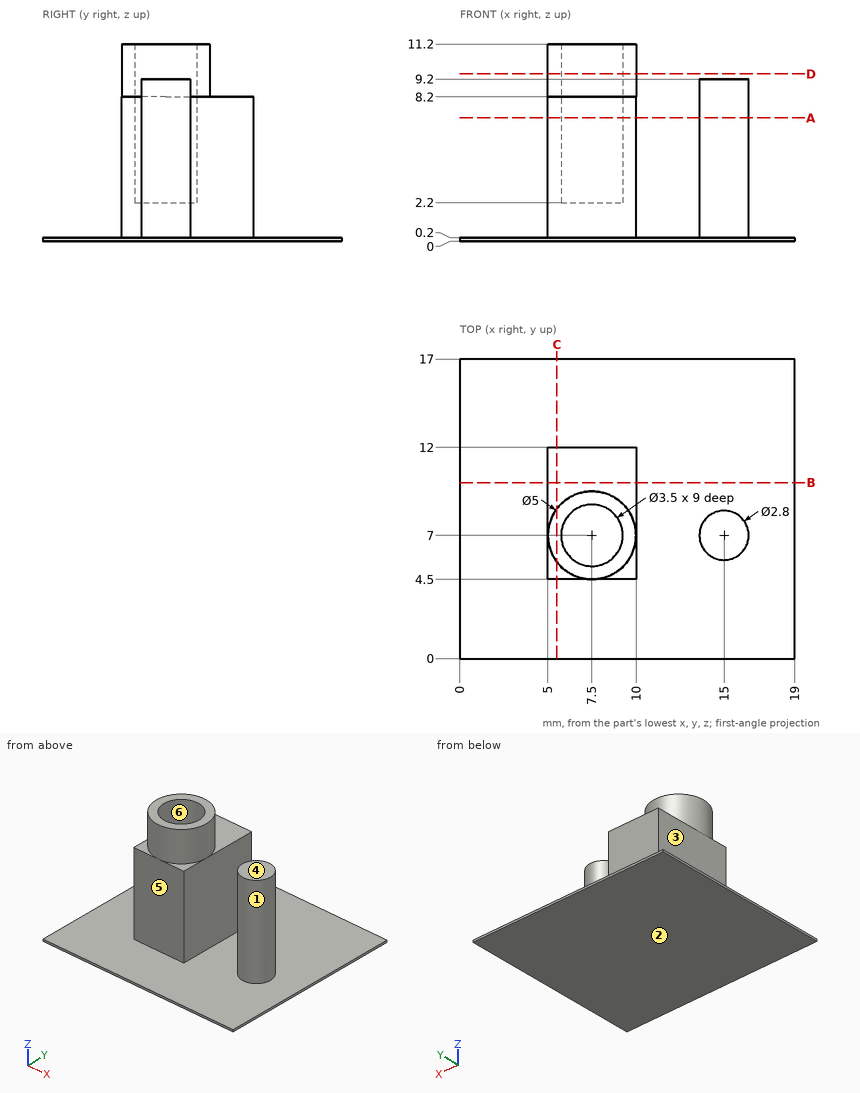
Could you check a few things on this drawing? It's one solid part, dimensions in mm from its lowest x, y, z. A direction names the side the tool comes from. Round coordinates to 2 decimals unless told otherwise and drop trailing zeros. Loops run counter-clockwise (first coordinate to the right, second up) from the corner with the lowest first, then second, coordinate; pieces in that order, holes last. Notation, with made-up numbers: M 50,68.25 L 107,68.25 A19 cw 107,73.25 Z; hole C 18,67 d5. An arc over 180 degrees is marked long. Write each question's results on one line, items separated by ' | '. Start each with the question number.
(1) If I drill on probe 1 along Y at (x, z) = (7.5, 7); probe 2 along Z at (x, y) = (5.75, 9.25); probe 3 along Z at (x, y) = (6.75, 2.25), over which ranges is the centre line in solid material (lowest first)? Write a range as from..to.
(2) I want a section at D-D (z = 9.5). Please give me the cut outline in (x, y), then the cut area to 3 significant figures.
(3) I want a section at B-B (y = 10). Please give me the cut outline in (x, z), then the cut area to 3 significant figures.
(4) Thinking about a two-plate mould opening in X: for the marked faces 1, 2 and 3, which applies, pulls with the +X half, pulls with the -X half, needs draft (parallel to the pull), parting line crosses it, or undercut?
(5) I want a section at C-C (x = 5.5). Please give me the cut outline in (y, z), then the cut area to 3 significant figures.
(6) I want a section at A-A (z = 7). Please give me the cut outline in (x, y), then the cut area to 3 significant figures.
(7) On a 3-axis mill with a long thin cutter (end or side, diameter ignored), from which of +Z, -Z, +X, -X, +Y, -Y can I reach the whole of each face in a straight line? I mean the marked faces 4, 5 and 6. Say none if no direction works.
(8) Will these pins go through, and if not, where does the flat tip stop? P1, Ø5, axis at x = 4, z = 3.5, coming from the -Y side; P2, Ø3, axis at y = 14, z = 3.5, coming from the +X side; P3, Ø1.5, axis at x = 7.5, z = 3, coming from the +Y side; P4, Ø2, axis at y = 8.5, z = 6, coming from the -X side.
Solved:
1) probe 1: y = 4.5..5.25, 8.75..12 | probe 2: z = 0..8.2 | probe 3: z = 0..0.2
2) outline: C 7.5,7 d5; hole C 7.5,7 d3.5 | area: 10.0 mm²
3) outline: M 0,0 L 19,0 L 19,0.2 L 10,0.2 L 10,8.2 L 5,8.2 L 5,0.2 L 0,0.2 Z | area: 43.8 mm²
4) face 1: undercut | face 2: needs draft | face 3: pulls with the -X half
5) outline: M 0,0 L 17,0 L 17,0.2 L 12,0.2 L 12,8.2 L 8.5,8.2 L 8.5,11.2 L 5.5,11.2 L 5.5,8.2 L 4.5,8.2 L 4.5,0.2 L 0,0.2 Z | area: 72.4 mm²
6) outline: M 5,4.5 L 10,4.5 L 10,12 L 5,12 Z; C 15,7 d2.8; hole C 7.5,7 d3.5 | area: 34.0 mm²
7) face 4: +Z, +X, +Y, -Y | face 5: +Z, +X, -X, -Y | face 6: +Z
8) P1: stops at y = 4.5 | P2: passes through | P3: stops at y = 12 | P4: stops at x = 5
